Verification items for the finished model (mm, model axes). A direction names the side the tool comes from. Give positions to 0.01 mm unless a question says otherwise; leave off trailing zeros. Order: outer loops, then holes, each group sorted by start corner. A loop starts at its lowest first (then second) coordinate and runs counter-clockwise, first axis right, second up.
Autodesk Fusion 360 part; units mm, degrees
sketch "Sketch1" plane through (0, 0, 0) normal (0, 0, 1) x (1, 0, 0)
  line L0 (0, 0) -> (153.4, 0)
  line L1 (153.4, 0) -> (153.4, -39.1)
  line L2 (153.4, -39.1) -> (0, -39.1)
  line L3 (0, -39.1) -> (0, 0)
  line L4 (-9.5, 9.5) -> (162.9, 9.5)
  line L5 (162.9, 9.5) -> (162.9, -48.6)
  line L6 (162.9, -48.6) -> (-9.5, -48.6)
  line L7 (-9.5, -48.6) -> (-9.5, 9.5)
  circle A0 centre (-4.5, 4.5) radius 1.7
  circle A1 centre (-4.5, -43.6) radius 1.7
  circle A2 centre (-4.5, -43.6) radius 3
  circle A3 centre (-4.5, 4.5) radius 3
  circle A4 centre (157.9, 4.5) radius 1.7
  circle A5 centre (157.9, 4.5) radius 3
  circle A6 centre (157.9, -43.6) radius 1.7
  circle A7 centre (157.9, -43.6) radius 3
  dimension "d1" = 153.4
  dimension "d2" = 39.1
  dimension "d3" = 172.4
  dimension "d4" = 58.1
  dimension "d5" = 9.5
  dimension "d6" = 9.5
  dimension "d7" = 3.4
  dimension "d8" = 5
  dimension "d9" = 5
  dimension "d10" = 3.4
  dimension "d11" = 5
  dimension "d12" = 5
  dimension "d13" = 6
  dimension "d14" = 6
  dimension "d15" = 3.4
  dimension "d16" = 5
  dimension "d17" = 5
  dimension "d18" = 6
  dimension "d19" = 3.4
  dimension "d20" = 5
  dimension "d21" = 5
  dimension "d22" = 6
extrude "Extrude1" add sketch "Sketch1" along normal blind 9.9 from surface at 3.1 contours A2 | A3 | A5 | A7 makes body 1 at (-1.5037, 4.3505, 9.7) makes body 2 at (160.1981, 6.4284, 9.7) makes body 3 at (-1.5037, -43.7495, 9.7) makes body 4 at (159.9947, -41.4524, 9.7)
extrude "Extrude2" add sketch "Sketch1" along normal blind 13 contours L4 L5 L6 L7 bodies 1 2 3 4
extrude "Extrude3" add sketch "Sketch1" along normal blind 3 contours L0 L1 L2 L3 bodies 1
sketch "Sketch2" plane through (0, 0, 13) normal (0, 0, 1) x (-1, 0, 0)
  circle A0 centre (4.5, -4.5) radius 1.7
  circle A1 centre (-157.9, 43.6) radius 1.7
  line L0 (-153.4, 39.1) -> (0, 39.1)
  line L1 (0, 39.1) -> (0, 0)
  line L2 (0, 0) -> (-153.4, 0)
  line L3 (-153.4, 0) -> (-153.4, 39.1)
  line L4 (9.5, 48.6) -> (-162.9, 48.6)
  line L5 (-162.9, 48.6) -> (-162.9, -9.5)
  line L6 (-162.9, -9.5) -> (9.5, -9.5)
  line L7 (9.5, -9.5) -> (9.5, 48.6)
  circle A2 centre (-157.9, -4.5) radius 1.7
  circle A3 centre (4.5, 43.6) radius 1.7
  line L8 (-20.386, -9.5) -> (-38.886, -9.5)
  line L9 (-38.886, -9.5) -> (-38.886, 0)
  line L10 (-38.886, 0) -> (-20.386, 0)
  line L11 (-20.386, 0) -> (-20.386, -9.5)
  dimension "d30" = 18.5
  dimension "d31" = 29.886
extrude "Extrude4" cut sketch "Sketch2" against normal blind 7.5 contours L2 L6 L8 L9 L10 L11 bodies 1
fillet "Fillet1" radius 5 4 edges at (-9.5, -48.6, 6.5) (-9.5, 9.5, 6.5) (162.9, 9.5, 6.5) (162.9, -48.6, 6.5) on bodies 1
(1) Section check C-C, the plane x = 29.5. Enter the section's corners in (y, z), then the cut area to 3 significant figures.
Solved:
outline: (-48.6, 0) - (9.5, 0) - (9.5, 5.5) - (0, 5.5) - (0, 3) - (-39.1, 3) - (-39.1, 13) - (-48.6, 13) - close
area: 293 mm2
(2) Go/stop test with flat-tipped pins: pin 1 (5 mm diameter, centred on x = 158, y = -43.5, fed in from -Z); pin 2 (1.5 mm diameter, centred on x = 16, y = -27, fed in from +Z); pin 3 (3 mm diameter, centred on x = 157.9, y = -43.6, fed in from +Z); pin 4 (2 mm diameter, centred on x = 36, z = 8, fed in from +Y). Record where each tip stops, or that it passes through.
Solved:
pin 1: stops at z = 3.1
pin 2: stops at z = 3
pin 3: passes through
pin 4: stops at y = -39.1
(3) Section check A-A, the plane z = 8.75. Enter the section's corners in (x, y).
Solved:
outline: (-9.5, -43.6) arc R5 ccw to (-4.5, -48.6) - (157.9, -48.6) arc R5 ccw to (162.9, -43.6) - (162.9, 4.5) arc R5 ccw to (157.9, 9.5) - (38.89, 9.5) - (38.89, 0) - (153.4, 0) - (153.4, -39.1) - (0, -39.1) - (0, 0) - (20.39, 0) - (20.39, 9.5) - (-4.5, 9.5) arc R5 ccw to (-9.5, 4.5) - close; hole circle Ø3.4 at (-4.5, -43.6); hole circle Ø3.4 at (-4.5, 4.5); hole circle Ø3.4 at (157.9, -43.6); hole circle Ø3.4 at (157.9, 4.5)
(4) Release check for a two-part mould opening along Y. For faces 1 (the flat face through (20.386, 5, 9)), 2 (the cylindrical face through (161.4, -47.17, 6.59)), 3 (the cylindrical face through (156.2, 4.43, 7.98)) record: pulls with the +Y half, pulls with the -Y half, needs draft (parallel to the pull), parting line crosses it, or undercut.
Solved:
face 1: needs draft
face 2: pulls with the -Y half
face 3: undercut
(5) Section check B-B, the plane y = -15. Enter the section's corners in (x, z).
Solved:
outline: (-9.5, 0) - (162.9, 0) - (162.9, 13) - (153.4, 13) - (153.4, 3) - (0, 3) - (0, 13) - (-9.5, 13) - close
(6) Set-up check for faces 4 (the flat face through (0, -20, 8)), 5 (the cylindrical face through (156.2, -43.67, 7.98)), 6 (the cylindrical face through (-5.15, -40.67, 1.53)): record each of +Z, -Z, +X, -X, +Y, -Y from which the full face is reachable in a straight line by a thin tool's end or side.
Solved:
face 4: +Z
face 5: +Z, -Z
face 6: -Z
(7) Scan lines: line 1 (Y direction, x = -4.5, z = 1.55); line 2 (Y direction, x = 105, z = 5.25); line 3 (X direction, y = -36.5, z = 3.75). Record each from-to range of solid material in increasing order.
Solved:
line 1: y = -48.6 to -46.6, -40.6 to 1.5, 7.5 to 9.5
line 2: y = -48.6 to -39.1, 0 to 9.5
line 3: x = -9.5 to 0, 153.4 to 162.9
